from build123d import *

# Parameters (mm, degrees)
CYLINDER017_R             = 2
CYLINDER017_DEPTH         = 9.2
CYLINDER018_R             = 3.5
CYLINDER018_DEPTH         = 10
CYLINDER016_R             = 2
CYLINDER016_DEPTH         = 9.2
CYLINDER019_R             = 3.5
CYLINDER019_DEPTH         = 10
CYLINDER014_R             = 2
CYLINDER014_DEPTH         = 9.2
CYLINDER015_R             = 3.5
CYLINDER015_DEPTH         = 10
CYLINDER013_R             = 2
CYLINDER013_DEPTH         = 9.2
CYLINDER012_R             = 3.5
CYLINDER012_DEPTH         = 10
BOX_W                     = 53
BOX_H                     = 62
BOX_DEPTH                 = 2
FILLET001_R               = 3
PAD003_DEPTH              = 40
FILLET004_R               = 3
FILLET005_R               = 1
FILLET002_R               = 5
FILLET003_R               = 3
FILLET003_PLACEMENT_ANGLE = 90


with BuildPart() as pass_screw_thread003:
    # Cylinder017 → Cylinder017 (new body)
    with BuildSketch(Plane.XY.offset(-9.2)):
        Circle(CYLINDER017_R)
    extrude(amount=CYLINDER017_DEPTH)


with BuildPart() as pass_screw_head003:
    # Cone007 → Cone007 (revolve)
    with BuildSketch(Plane.XZ):
        Polygon((0, 0), (2, 0), (3.5, 3.4), (0, 3.4), align=None)
    revolve(axis=Axis((0, 0, 0), (0, 0, 1)))


with BuildPart() as pass_screw003:
    # Cylinder018 → Cylinder018 (new body)
    with BuildSketch(Plane.XY.offset(3.2)):
        Circle(CYLINDER018_R)
    extrude(amount=CYLINDER018_DEPTH)

    # Fusion016: union pass-screw-thread003, pass-screw-head003
    add(pass_screw_thread003.part)
    add(pass_screw_head003.part)


with BuildPart() as pass_screw003_1:
    # Fusion016 placement: moved
    add(pass_screw003.part.moved(Location((42, 0, 18))))


with BuildPart() as pass_screw_thread002:
    # Cylinder016 → Cylinder016 (new body)
    with BuildSketch(Plane.XY.offset(-9.2)):
        Circle(CYLINDER016_R)
    extrude(amount=CYLINDER016_DEPTH)


with BuildPart() as pass_screw_head002:
    # Cone006 → Cone006 (revolve)
    with BuildSketch(Plane.XZ):
        Polygon((0, 0), (2, 0), (3.5, 3.4), (0, 3.4), align=None)
    revolve(axis=Axis((0, 0, 0), (0, 0, 1)))


with BuildPart() as pass_screw_top:
    # Cylinder019 → Cylinder019 (new body)
    with BuildSketch(Plane.XY.offset(3.2)):
        Circle(CYLINDER019_R)
    extrude(amount=CYLINDER019_DEPTH)

    # Fusion015: union pass-screw-thread002, pass-screw-head002
    add(pass_screw_thread002.part)
    add(pass_screw_head002.part)


with BuildPart() as pass_screw_top_1:
    # Fusion015 placement: moved
    add(pass_screw_top.part.moved(Location((-5, 0, 18))))

    # Fusion017: union pass-screw003
    add(pass_screw003_1.part)


with BuildPart() as pass_screw_top_2:
    # Fusion017 placement: moved
    add(pass_screw_top_1.part.moved(Location((0, 56, 0))))


with BuildPart() as pass_screw_thread001:
    # Cylinder014 → Cylinder014 (new body)
    with BuildSketch(Plane.XY.offset(-9.2)):
        Circle(CYLINDER014_R)
    extrude(amount=CYLINDER014_DEPTH)


with BuildPart() as pass_screw_head001:
    # Cone005 → Cone005 (revolve)
    with BuildSketch(Plane.XZ):
        Polygon((0, 0), (2, 0), (3.5, 3.4), (0, 3.4), align=None)
    revolve(axis=Axis((0, 0, 0), (0, 0, 1)))


with BuildPart() as pass_screw001:
    # Cylinder015 → Cylinder015 (new body)
    with BuildSketch(Plane.XY.offset(3.2)):
        Circle(CYLINDER015_R)
    extrude(amount=CYLINDER015_DEPTH)

    # Fusion013: union pass-screw-thread001, pass-screw-head001
    add(pass_screw_thread001.part)
    add(pass_screw_head001.part)


with BuildPart() as pass_screw001_1:
    # Fusion013 placement: moved
    add(pass_screw001.part.moved(Location((42, 0, 18))))


with BuildPart() as pass_screw_thread:
    # Cylinder013 → Cylinder013 (new body)
    with BuildSketch(Plane.XY.offset(-9.2)):
        Circle(CYLINDER013_R)
    extrude(amount=CYLINDER013_DEPTH)


with BuildPart() as pass_screw_head:
    # Cone → Cone (revolve)
    with BuildSketch(Plane.XZ):
        Polygon((0, 0), (2, 0), (3.5, 3.4), (0, 3.4), align=None)
    revolve(axis=Axis((0, 0, 0), (0, 0, 1)))


with BuildPart() as fusion018:
    # Cylinder012 → Cylinder012 (new body)
    with BuildSketch(Plane.XY.offset(3.2)):
        Circle(CYLINDER012_R)
    extrude(amount=CYLINDER012_DEPTH)

    # Fusion012: union pass-screw-thread, pass-screw-head
    add(pass_screw_thread.part)
    add(pass_screw_head.part)


with BuildPart() as fusion018_1:
    # Fusion012 placement: moved
    add(fusion018.part.moved(Location((-5, 0, 18))))

    # Fusion014: union pass-screw001
    add(pass_screw001_1.part)

    # Fusion018: union pass-screw-top
    add(pass_screw_top_2.part)


with BuildPart() as top_plate_with_screws:
    # Box → Box (new body)
    with BuildSketch(Plane(origin=(-8, -3, 16.6), x_dir=(1, 0, 0), z_dir=(0, 0, 1))):
        with Locations((26.5, 31)):
            Rectangle(BOX_W, BOX_H)
    extrude(amount=BOX_DEPTH)

    # Fillet001
    fillet001_edges = [top_plate_with_screws.edges().sort_by_distance(p)[0] for p in [
        (-8, -3, 17.6),
        (-8, 59, 17.6),
        (45, -3, 17.6),
        (45, 59, 17.6),
    ]]
    fillet(fillet001_edges, radius=FILLET001_R)

    # Cut002: cut Fusion018
    add(fusion018_1.part, mode=Mode.SUBTRACT)


with BuildPart() as final_top_plate_with_clip:
    # Sketch003 → Pad003 (new body)
    with BuildSketch(Plane.XY):
        Polygon((0, 0), (30.749545, 0), (30.749545, 2), (29.374773, 5), (25.374773, 5), (24, 2), (2, 2), (2, 17.5), (24, 17.5), (25.374773, 14.5), (29.374773, 14.5), (30.749545, 17.5), (30.749545, 19.5), (0, 19.5), align=None)
    extrude(amount=PAD003_DEPTH)

    # Fillet004
    fillet004_edges = [final_top_plate_with_clip.edges().sort_by_distance(p)[0] for p in [
        (29.374773, 5, 20),
        (29.374773, 14.5, 20),
    ]]
    fillet(fillet004_edges, radius=FILLET004_R)

    # Fillet005
    fillet005_edges = [final_top_plate_with_clip.edges().sort_by_distance(p)[0] for p in [
        (30.749545, 2, 20),
        (30.749545, 0, 20),
        (30.749545, 19.5, 20),
        (30.749545, 17.5, 20),
    ]]
    fillet(fillet005_edges, radius=FILLET005_R)

    # Fillet002
    fillet002_edges = [final_top_plate_with_clip.edges().sort_by_distance(p)[0] for p in [
        (2, 2, 20),
        (2, 17.5, 20),
    ]]
    fillet(fillet002_edges, radius=FILLET002_R)

    # Fillet003
    fillet003_edges = [final_top_plate_with_clip.edges().sort_by_distance(p)[0] for p in [
        (0, 0, 20),
        (0, 19.5, 20),
    ]]
    fillet(fillet003_edges, radius=FILLET003_R)


with BuildPart() as final_top_plate_with_clip_1:
    # Fillet003 placement: moved
    add(final_top_plate_with_clip.part.moved(Location((-8, 48, 18))).rotate(Axis((-8, 48, 18), (1, 0, 0)), FILLET003_PLACEMENT_ANGLE))

    # Fusion019: union top-plate-with-screws
    add(top_plate_with_screws.part)


with BuildPart() as final_top_plate_with_clip_2:
    # Fusion019 placement: moved
    add(final_top_plate_with_clip_1.part.moved(Location((-37, 0, -16.6))))


solid = final_top_plate_with_clip_2.part
Geometry: final body of the model. Coordinates: model frame, mm. A direction names the side the tool comes from. Coordinates: 2 decimals unless noted, no trailing zeros. Loops run counter-clockwise (first coordinate to the right, second up) from the corner with the lowest first, then second, coordinate; pieces in that order, holes last. Notation, with made-up numbers: M 14.5,65 L 40.5,65 A13 cw 40.5,89 Z; hole C 54,26 d7. An arc over 180 degrees is marked long. One line per item, written item: value. Start each with the question number.
1) Pin query (flat end, axial travel): P1, Ø3, axis at y = 29.5, z = 10.5, coming from the +X side; P2, Ø6, axis at x = -11.5, z = 19, coming from the +Y side; P3, Ø3, axis at x = 5, y = 56, coming from the +Z side; P4, Ø5, axis at x = -28.5, y = 33, coming from the -Z side. Return the tip coordinate at first contact, or that it passes through.
2) Cut plane C-C (z = 5.5). Return loops of the section in (x, y).
3) Cut plane B-B (y = 9.5). Return loops of the section in (x, z), then the cut area to 3 significant figures.
4) Cut plane D-D (x = -4). Return loops of the section in (y, z), then the cut area to 3 significant figures.
5) Draft query along Y for faces 1 (the flat face through (-20.32, 28.28, 17.42)), 2 (the flat face through (-19, 59, 1)), 3 (the cylindrical face through (-44, 0, 1)), 4 (the cylindrical face through (7.1, -2.14, 1.01)). Return one class per face: released by +Y, released by -Y, zero draft, split by the parting line, or undercut.
6) Cut plane A-A (x = -22.5). Return loops of the section in (y, z), then the cut area to 3 significant figures.
7) Material intervals for L1, parallel to Y at x = -42, z = 0.7; L2, parallel to X at y = 0, z = 1.1; L3, parallel to Z at x = -23.5, y = 24.5, sorted ascending. Write a range as from..to.
8) Reachability of faces 5 (the cylindrical face through (-41.5, 27.72, 4.83)), 6 (the flat face through (-30.8, 48, 19.2)), 7 (the flat face through (-19, 28, 0)) from +Z, -Z, +X, -X, +Y, -Y: full face, straight path, thin tool, end or side. Return the list, or none.
Evaluation:
1. P1: x = -43
1. P2: y = 48
1. P3: through
1. P4: z = 0
2. outline: M -45,8 L -42.07,8 L -42.07,48 L -45,48 Z; M -20.04,8 L -15.41,8 L -15.41,48 L -20.04,48 Z
3. outline: M -45,0 L 8,0 L 8,2 L -14.33,2 A1 ccw -14.25,2.4 L -14.25,3.18 A1 ccw -14.34,3.6 L -14.82,4.65 A3 ccw -17.55,6.4 L -19.63,6.4 L -21,3.4 L -38,3.4 A5 cw -43,8.4 L -43,13.9 A5 cw -38,18.9 L -21,18.9 L -19.63,15.9 L -17.55,15.9 A3 ccw -14.82,17.65 L -14.34,18.7 A1 ccw -14.25,19.12 L -14.25,19.9 A1 ccw -15.25,20.9 L -42,20.9 A3 ccw -45,17.9 L -45,4.4 A3 ccw -43.8,2 L -45,2 Z
3. area: 280 mm^2
4. outline: M -3,0 L 59,0 L 59,2 L -3,2 Z
4. area: 124 mm^2
5. face 1: zero draft
5. face 2: released by +Y
5. face 3: undercut
5. face 4: released by -Y
6. outline: M -3,0 L 59,0 L 59,2 L 48,2 L 48,3.4 L 8,3.4 L 8,2 L -3,2 Z; M 8,18.9 L 48,18.9 L 48,20.9 L 8,20.9 Z
6. area: 260 mm^2
7. L1: -3..-2, 2..54, 58..59
7. L2: -45..-44, -40..3, 7..8
7. L3: 0..3.4, 18.9..20.9
8. face 5: +Y, -Y
8. face 6: +Z, +X, -X, +Y
8. face 7: -Z, +X, -X, +Y, -Y
